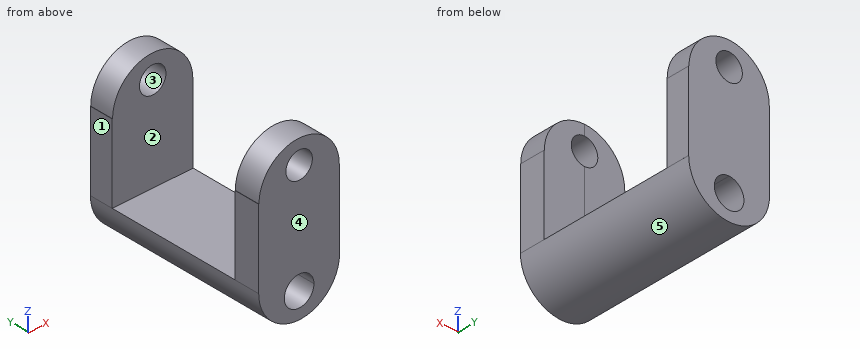
from build123d import *

# Parameters (mm, degrees)
F0_R          = 7.3981618973
F1_DEPTH      = 50.8
F1_DEPTH_BACK = 50.8
F2_W          = 74.1309896111
F2_H          = 66.0332143307
F3_DEPTH      = 25.4
F3_DEPTH_BACK = 25.4


# Not quite as in the source:
# - the program builds the solid bodies; features that only make, move or delete a surface that nothing else refers to are left out


with BuildPart() as f1:
    # F0 (on Front) → F1 (new body, two sides)
    with BuildSketch(Plane.XZ) as f1_sk:
        with BuildLine():
            Line((-22.5902460515, 0), (-22.5853170946, 0))
            ThreePointArc((-22.5853170946, 0), (0, -22.5853170946), (22.5853170946, 0))
            Line((22.5853170946, 0), (22.5902460515, 0))
            Line((22.5902460515, 0), (22.5902460515, 43.5050576925))
            Line((22.5902460515, 43.5050576925), (22.4241250182, 43.5050576925))
            ThreePointArc((22.4241250182, 43.5050576925), (0, 65.9291827108), (-22.4241250182, 43.5050576925))
            Line((-22.4241250182, 43.5050576925), (-22.5902460515, 43.5050576925))
            Line((-22.5902460515, 43.5050576925), (-22.5902460515, 0))
        make_face()
        with BuildLine():
            ThreePointArc((0, -0.2681852946), (5.848754541, -2.6908187485), (8.2713879948, -8.5395732895))
            ThreePointArc((8.2713879948, -8.5395732895), (-5.848754541, -14.3883278304), (0, -0.2681852946))
        make_face(mode=Mode.SUBTRACT)
        with Locations((0, 52.7734495699)):
            Circle(F0_R, mode=Mode.SUBTRACT)
    extrude(amount=F1_DEPTH)
    extrude(f1_sk.sketch, amount=-F1_DEPTH_BACK)

    # F2 (on Right) → F3 (cut, two sides)
    with BuildSketch(Plane.YZ) as f3_sk:
        with Locations((0.5546920002, 33.0166071653)):
            Rectangle(F2_W, F2_H)
    extrude(amount=-F3_DEPTH, mode=Mode.SUBTRACT)
    extrude(f3_sk.sketch, amount=F3_DEPTH_BACK, mode=Mode.SUBTRACT)


solid = f1.part
Build history of the part. All positions in model axes, mm. Face numbers are marked on the shaded views. A direction names the side the tool comes from. Round coordinates to 2 decimals unless told otherwise and drop trailing zeros. Write each loop counter-clockwise with the first axis right and the second up, starting at its lowest first coordinate (ties: lowest second). Pieces come first, ordered by that corner, then holes. Notation, with made-up numbers: M 60.25,18 L 65.25,18 A19 cw 65.25,37 Z; hole C 72,-20.5 d2. An arc over 180 degrees is marked long. Answer in a Markdown table with one row per item.
1. Probe L1, parallel to Z at x = 0, y = 44; L2, parallel to Z at x = 0, y = -31; L3, parallel to Y at x = -13, z = 25. List the from-to ranges inside material, lowest first. Write a range as [from, to].
Geometry check:
| item | result |
|---|---|
| L1 | [-22.59, -16.81], [-0.27, 45.38], [60.17, 65.93] |
| L2 | [-22.59, -16.81], [-0.27, 0] |
| L3 | [-50.8, -36.51], [37.62, 50.8] |
2. Which spindle directions (+Z, -Z, +X, -X, +Y, -Y) get a long thin tool onto all of the face, cutting with end or side? Do the marked faces 1 and 2. Say none if no direction does.
Geometry check:
| item | result |
|---|---|
| face 1 | +Z, -Z, -X, +Y, -Y |
| face 2 | +Z, +X, -X |
3. Saw through at C-C (z = 56). List the corners of the cut face in (x, y), and give its area (3 significant figures).
Geometry check:
| item | result |
|---|---|
| outline | M -18.62,-50.8 L -6.66,-50.8 L -6.66,-36.51 L -18.62,-36.51 Z; M -18.62,37.62 L -6.66,37.62 L -6.66,50.8 L -18.62,50.8 Z; M 6.66,-50.8 L 18.62,-50.8 L 18.62,-36.51 L 6.66,-36.51 Z; M 6.66,37.62 L 18.62,37.62 L 18.62,50.8 L 6.66,50.8 Z |
| area | 657 mm2 |
4. Saw through at D-D (y = 12). List the corners of the cut face in (x, z), and give its area (3 significant figures).
Geometry check:
| item | result |
|---|---|
| outline | M -22.59,0 A22.59 ccw 22.59,0 Z; hole C 0,-8.54 d16.54 |
| area | 586 mm2 |
5. Mould opens along X. For the marked faces 3, 4 and 5 say: +X half, -X half, draft (parallel to the pull), parting line (faces both ways), or undercut.
Geometry check:
| item | result |
|---|---|
| face 3 | undercut |
| face 4 | draft |
| face 5 | parting line |
6. Saw through at A-A (z = 40). List the corners of the cut face in (x, y), and give its area (3 significant figures).
Geometry check:
| item | result |
|---|---|
| outline | M -22.59,-50.8 L 22.59,-50.8 L 22.59,-36.51 L -22.59,-36.51 Z; M -22.59,37.62 L 22.59,37.62 L 22.59,50.8 L -22.59,50.8 Z |
| area | 1,240 mm2 |
7. Saw through at B-B (x = 4.5). List the corners of the cut face in (y, z), and give its area (3 significant figures).
Geometry check:
| item | result |
|---|---|
| outline | M -50.8,-22.13 L 50.8,-22.13 L 50.8,-15.48 L -50.8,-15.48 Z; M -50.8,-1.6 L 50.8,-1.6 L 50.8,46.9 L 37.62,46.9 L 37.62,0 L -36.51,0 L -36.51,46.9 L -50.8,46.9 Z; M -50.8,58.65 L -36.51,58.65 L -36.51,65.47 L -50.8,65.47 Z; M 37.62,58.65 L 50.8,58.65 L 50.8,65.47 L 37.62,65.47 Z |
| area | 2,310 mm2 |
8. Flat gauge pins, fed straight in: P1, Ø12, axis at y = 32, z = 49, coming from the -X side; P2, Ø10, axis at x = -16.5, y = 16.5, coming from the +Z side; P3, Ø1, axis at x = 8.5, y = -23, coming from the -Z side. Where does each tip first touch, or does it go through?
Geometry check:
| item | result |
|---|---|
| P1 | x = -22.17 |
| P2 | z = 0 |
| P3 | z = -21.12 |
